Build history of the part. All positions in model axes, mm. Face numbers are marked on the shaded views. A direction names the side the tool comes from. Round coordinates to 2 decimals unless told otherwise and drop trailing zeros. Write each loop counter-clockwise with the first axis right and the second up, starting at its lowest first coordinate (ties: lowest second). Pieces come first, ordered by that corner, then holes.
Item 1: 3-axis set-ups, long thin cutter, end or side, ignore diameter. For the marked faces 5 and 6: which of +Z, -Z, +X, -X, +Y, -Y reach the whole face in a straight line?
Item 2: Wall check: probe 1 along X at (y, z) = (-4, 14); probe 2 along Y at (x, z) = (-22, 13.1); probe 3 along Y at (x, z) = (-28, 20). Give the ranges that are in metal, low to high.
Item 3: Band-saw the part on B-B, the plane x = -22. Count the separate pieces of the cut face and the enclosed holes in it, then the cut area to 3 significant figures.
Item 4: Band-saw the part on C-C, the plane x = -12. Write the cut outline in (y, z).
Item 5: Mould opens along Z. For the marked faces 1, 2, 3 and 4 say: +Z half, -Z half, draft (parallel to the pull), parting line (faces both ways), or undercut.
Item 6: Band-saw the part on A-A, the plane z = 18.5. Write the cut outline in (x, y), then the cut area to 3 significant figures.
Item 7: Drop flat-ended pins along their axis: pin 1 Ø12 at (x, z) = (-17.5, 35.5) entering from +Y; pin 2 Ø1.5 at (x, y) = (-25, -2.5) entering from -Z; pin 3 Ø3.5 at (x, y) = (-22, 4) entering from +Z; pin 4 Ø4 at (y, z) = (-5.5, 8.5) entering from -X. Give the stop position or say it passes through.
```python
from build123d import *

# Parameters (mm, degrees)
SKETCH040_R  = 1.5
PAD029_DEPTH = 20
SKETCH045_R  = 3
PAD031_DEPTH = 10
SKETCH037_W  = 15.25
SKETCH037_H  = 2.793113
SKETCH038_W  = 8.25
SKETCH038_H  = 8.85529
PAD030_DEPTH = 4


with BuildPart() as mountingblock_cutout:
    # Sketch042 → Loft002 section 0
    with BuildSketch(Plane.YZ.offset(16.5)):
        Polygon((15.5, 0), (7.75, 13.423394), (-7.75, 13.423394), (-15.5, 0), (-7.75, -13.423394), (7.75, -13.423394), align=None)
    # Sketch043 → Loft002 section 1
    with BuildSketch(Plane.YZ.offset(31.5)):
        Polygon((8.5, 0), (4.25, 7.361216), (-4.25, 7.361216), (-8.5, 0), (-4.25, -7.361216), (4.25, -7.361216), align=None)
    loft(ruled=True)


with BuildPart() as screw_cutouts:
    # Sketch040 → Pad029 (new body)
    with BuildSketch(Plane.XY.offset(16)):
        with Locations((22, 4)):
            Circle(SKETCH040_R)
        with Locations((22, -4)):
            Circle(SKETCH040_R)
    extrude(amount=-PAD029_DEPTH)


with BuildPart() as cutouts:
    # Sketch045 → Pad031 (new body)
    with BuildSketch(Plane.XY.offset(16)):
        with Locations((22, 4)):
            Circle(SKETCH045_R)
        with Locations((22, -4)):
            Circle(SKETCH045_R)
    extrude(amount=PAD031_DEPTH)

    # Fusion004008: union MountingBlock Cutout, Screw Cutouts
    add(mountingblock_cutout.part)
    add(screw_cutouts.part)


with BuildPart() as mountingblock_mount:
    # Sketch037 → Loft001 section 0
    with BuildSketch(Plane.YZ.offset(16.5)):
        with Locations((0, 14.603444)):
            Rectangle(SKETCH037_W, SKETCH037_H)
    # Sketch038 → Loft001 section 1
    with BuildSketch(Plane.YZ.offset(31.5)):
        with Locations((0, 11.572355)):
            Rectangle(SKETCH038_W, SKETCH038_H)
    loft(ruled=True)


with BuildPart() as base_plate:
    # Sketch041 → Pad030 (new body)
    with BuildSketch(Plane.XZ.offset(8)):
        Polygon((31.289345, 0), (31.289345, 15.901777), (26.297165, 39.708817), (0, 39.708817), (0, 25.462919), (7.794133, 25.462919), (14.835288, 20.052349), (17.132925, 15.827662), (17.132925, 0), align=None)
    extrude(amount=-PAD030_DEPTH)

    # Fusion004009: union MountingBlock Mount
    add(mountingblock_mount.part)

    # Cut007003: cut cutouts
    add(cutouts.part, mode=Mode.SUBTRACT)


with BuildPart() as part_mirroring:
    # Part__Mirroring: instance of Base Plate
    add(base_plate.part.mirror(Plane(origin=(0, 0, 0), x_dir=(0, -1, 0), z_dir=(1, 0, 0))))


solid = part_mirroring.part
```
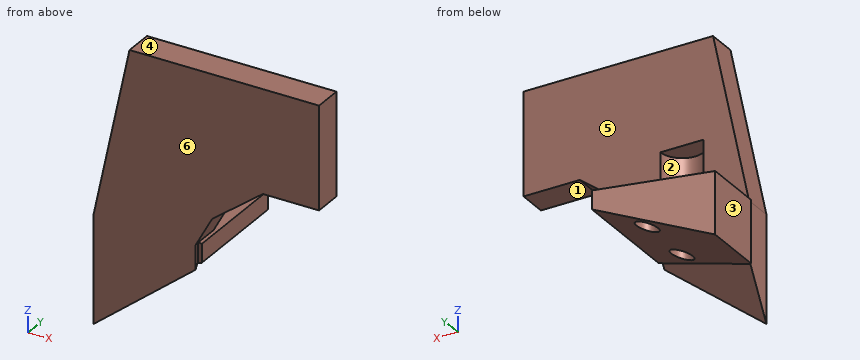
Results:
1. face 5: +Z, +X, -X, +Y
1. face 6: +Z, -Z, +X, -X, -Y
2. probe 1: x = -31.5 to -23.5, -20.5 to -16.5
2. probe 2: y = -8 to -5.5, -2.5 to 2.5, 5.5 to 6.34
2. probe 3: y = -8 to -4
3. separate pieces: 3
3. enclosed holes: 0
3. area: 107 mm2
4. outline: (-8, 22.23) - (-4, 22.23) - (-4, 39.71) - (-8, 39.71) - close
5. face 1: -Z half
5. face 2: undercut
5. face 3: draft
5. face 4: +Z half
6. outline: (-30.74, -8) - (-15.68, -8) - (-15.68, -4) - (-19, -4) arc R3 cw to (-25, -4) - (-30.74, -4) - close
6. area: 46.1 mm2
7. pin 1: stops at y = -4
7. pin 2: stops at z = 9.69
7. pin 3: stops at z = 16
7. pin 4: stops at x = -31.5
